```python
from build123d import *

# Parameters (mm, degrees)
SKETCH1_W           = 20
SKETCH1_H           = 20
BOSS_EXTRUDE1_DEPTH = 150
SKETCH2_W           = 7
SKETCH2_H           = 21
SKETCH2_W_2         = 21
SKETCH2_H_2         = 7
BOSS_EXTRUDE2_DEPTH = 2
BOSS_EXTRUDE3_DEPTH = 50
SKETCH4_R           = 15
CUT_EXTRUDE1_DEPTH  = 50


with BuildPart() as part:
    # Sketch1 → Boss-Extrude1 (new body)
    with BuildSketch(Plane.XY):
        Polygon((22.477189953, 38), (-22.477189953, 38), (-16.268065934, 16.268065934), (-38, 22.477189953), (-38, -22.477189953), (-16.268065934, -16.268065934), (-22.477189953, -38), (22.477189953, -38), (16.268065934, -16.268065934), (38, -22.477189953), (38, 22.477189953), (16.268065934, 16.268065934), align=None)
        Polygon((12.5, 14), (-12.5, 14), (-18.5, 35), (18.5, 35), align=None, mode=Mode.SUBTRACT)
        Rectangle(SKETCH1_W, SKETCH1_H, mode=Mode.SUBTRACT)
        Polygon((14, -12.5), (14, 12.5), (35, 18.5), (35, -18.5), align=None, mode=Mode.SUBTRACT)
        Polygon((-12.5, -14), (12.5, -14), (18.5, -35), (-18.5, -35), align=None, mode=Mode.SUBTRACT)
        Polygon((-14, 12.5), (-14, -12.5), (-35, -18.5), (-35, 18.5), align=None, mode=Mode.SUBTRACT)
    extrude(amount=BOSS_EXTRUDE1_DEPTH)

    # Sketch2 → Boss-Extrude2 (add)
    with BuildSketch(Plane.XY):
        with Locations((0, 24.5)):
            Rectangle(SKETCH2_W, SKETCH2_H)
        with Locations((24.5, 0)):
            Rectangle(SKETCH2_W_2, SKETCH2_H_2)
        with Locations((0, -24.5)):
            Rectangle(SKETCH2_W, SKETCH2_H)
        with Locations((-24.5, 0)):
            Rectangle(SKETCH2_W_2, SKETCH2_H_2)
    extrude(amount=BOSS_EXTRUDE2_DEPTH)

    # Sketch3 → Boss-Extrude3 (add)
    with BuildSketch(Plane.XY.offset(150)):
        Polygon((40, -22.477189953), (40, -15), (105, -15), (105, 15), (40, 15), (40, 22.477189953), (38, 22.477189953), (38, -22.477189953), align=None)
        Polygon((-38, 22.477189953), (-40, 22.477189953), (-40, 15), (-105, 15), (-105, -15), (-40, -15), (-40, -22.477189953), (-38, -22.477189953), align=None)
    extrude(amount=-BOSS_EXTRUDE3_DEPTH)

    # Sketch4 → Cut-Extrude1 (cut)
    with BuildSketch(Plane(origin=(0, 15, 0), x_dir=(1, 0, 0), z_dir=(0, 1, 0))):
        with Locations(Location((80, -125, 0), (0, 0, 270))):
            Circle(SKETCH4_R)
        with Locations(Location((-80, -125, 0), (0, 0, 270))):
            Circle(SKETCH4_R)
        with BuildLine():
            Line((80, -100), (80, -91.906284046))
            Line((80, -91.906284046), (116.237187359, -91.906284046))
            Line((116.237187359, -91.906284046), (116.237187359, -153.794533515))
            Line((116.237187359, -153.794533515), (80, -153.794533515))
            Line((80, -153.794533515), (80, -150))
            ThreePointArc((80, -150), (105, -125), (80, -100))
        make_face()
        with BuildLine():
            Line((-80, -153.794533515), (-80, -150))
            ThreePointArc((-80, -150), (-105, -125), (-80, -100))
            Line((-80, -100), (-80, -91.906284046))
            Line((-80, -91.906284046), (-116.237187359, -91.906284046))
            Line((-116.237187359, -91.906284046), (-116.237187359, -153.794533515))
            Line((-116.237187359, -153.794533515), (-80, -153.794533515))
        make_face()
    extrude(amount=-CUT_EXTRUDE1_DEPTH, mode=Mode.SUBTRACT)


solid = part.part
```
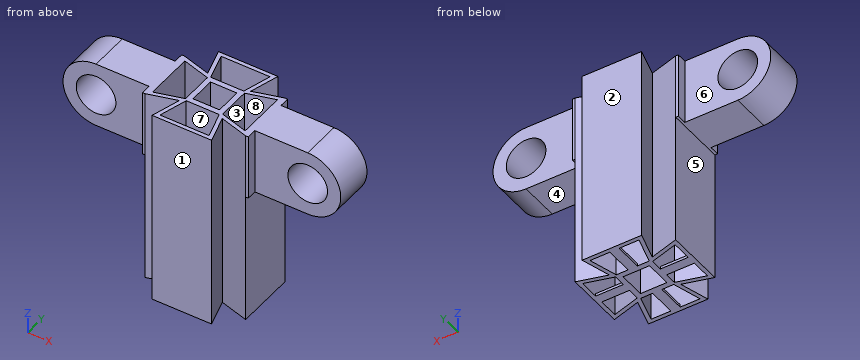
For this review, take the finished solid that the model builds, in its own axes (mm). Face numbers are marked on the shaded views. A direction names the side the tool comes from. Coordinates: 2 decimals unless noted, no trailing zeros. Order: outer loops, then holes, each group sorted by start corner. A loop starts at its lowest first (then second) coordinate and runs counter-clockwise, first axis right, second up. Notation, with made-up numbers: (72.5, 60.25) - (108.5, 60.25) arc R20 ccw to (108.5, 94.25) - close; hole circle Ø9 at (17, 34.25). An arc over 180 degrees is marked (long way). Answer as a JSON object with one key per item and string values. Group by question number.
1. Clearance check with flat-ended pins moving along their axes: P1, Ø1, axis at y = -26.5, z = 1, coming from the +X side; P2, Ø2, axis at x = -39, z = 124, coming from the -Y side; P3, Ø8, axis at y = -20, z = 129, coming from the +X side. State where each tip first meets the part, or that it passes through.
2. We need section C-C on x = -70. State the section outline as (y, z) points.
3. For the marked faces 4, 5, 6, 7 and 8, list the 3-axis set-ups (+Z, -Z, +X, -X, +Y, -Y) from which the entire face can be reached by the end or side of a thin tool; tool diameter is ignored.
4. The part is to be moulded in two halves that separate along Y. For the marked faces 1, 2 and 3, say which applies: pulls with the +Y half, pulls with the -Y half, needs draft (parallel to the pull), parting line crosses it, or undercut.
5. For probe 1 along X at (y, z) = (-6, 125); probe 2 along Y at (x, z) = (8.5, 24); probe 3 along Y at (x, z) = (-11, 111), list the stretches that pass through material, from the lowest coordinate up.
6. We need section B-B on z = 125. Give the number of separate pieces and of enclosed holes in the cut face, then the cut area to 3 significant figures.
7. We need section A-A on y = 7.5. State the section outline as (x, z) points.
Final values:
{
 "1": {"P1": "x = 19.33", "P2": "y = -22.48", "P3": "x = 40"},
 "2": {"outline": "(-15, 100) - (15, 100) - (15, 113.82) - (-15, 113.82) - close; (-15, 136.18) - (15, 136.18) - (15, 150) - (-15, 150) - close"},
 "3": {"face 4": "-Z, +X, +Y, -Y", "face 5": "-Z, -X, +Y, -Y", "face 6": "+Z, -Z, -X, +Y", "face 7": "+Z", "face 8": "+Z, -Z"},
 "4": {"face 1": "pulls with the -Y half", "face 2": "pulls with the +Y half", "face 3": "undercut"},
 "5": {"probe 1": "-105 to -95, -65 to -35, -14 to -10, 10 to 14, 35 to 65, 95 to 105", "probe 2": "-38 to -35, -14 to -10, 10 to 14, 35 to 38", "probe 3": "-38 to -35, -14 to 14, 35 to 38"},
 "6": {"separate pieces": "3", "enclosed holes": "5", "area": "3,700 mm²"},
 "7": {"outline": "(-80, 100) - (-38, 100) - (-38, 0) - (-35, 0) - (-35, 150) - (-80, 150) arc R25 ccw to start; (-14, 0) - (-10, 0) - (-10, 150) - (-14, 150) - close; (10, 0) - (14, 0) - (14, 150) - (10, 150) - close; (35, 0) - (38, 0) - (38, 100) - (80, 100) arc R25 ccw to (80, 150) - (35, 150) - close; hole circle Ø30 at (-80, 125); hole circle Ø30 at (80, 125)"}
}
